```python
from build123d import *

# Parameters (mm, degrees)
SKETCH1_R           = 4.45
BOSS_EXTRUDE1_DEPTH = 5.6
CHAMFER1_SIZE       = 0.6


with BuildPart() as part:
    # Sketch1 → Boss-Extrude1 (new body)
    with BuildSketch(Plane(origin=(0, 0, 0), x_dir=(1, 0, 0), z_dir=(0, 1, 0))):
        with BuildLine():
            Line((6, 10.392304845), (-6, 10.392304845))
            ThreePointArc((-6, 10.392304845), (-12, 0), (-6, -10.392304845))
            Line((-6, -10.392304845), (6, -10.392304845))
            ThreePointArc((6, -10.392304845), (12, 0), (6, 10.392304845))
        make_face()
        Circle(SKETCH1_R, mode=Mode.SUBTRACT)
    extrude(amount=BOSS_EXTRUDE1_DEPTH)

    # Chamfer1
    chamfer1_edges = [part.edges().sort_by_distance(p)[0] for p in [
        (-4.45, 5.6, 0),
    ]]
    chamfer(chamfer1_edges, length=CHAMFER1_SIZE)


solid = part.part
```
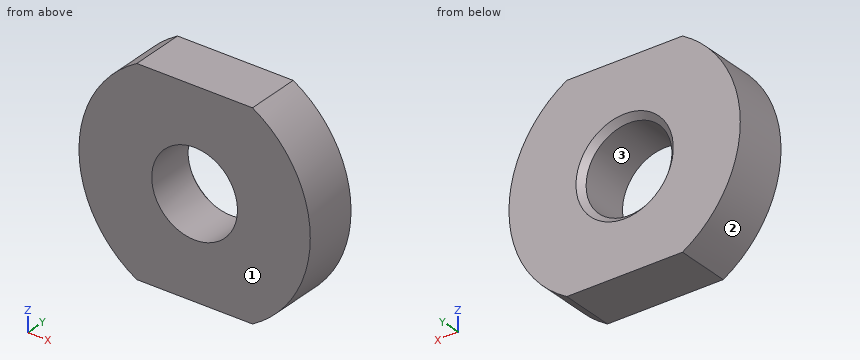
Geometry check sheet. Reference: the model listing, model coordinates, mm. Face numbers are marked on the shaded views. Round coordinates to 2 decimals unless told otherwise and drop trailing zeros. Order: outer loops, then holes, each group sorted by start corner. A loop starts at its lowest first (then second) coordinate and runs counter-clockwise, first axis right, second up. Notation, with made-up numbers: (68.5, -7) -> (96.5, -7) arc R23 cw to (96.5, 8) -> close; hole circle Ø9 at (68.25, -9). An arc over 180 degrees is marked (long way). Return JSON: item names as keys, results as strings. Group by question number.
Q1. Gauge pin test, flat ends, axial feed: pin 1 (1 mm diameter, centred on x = -9.5, z = -7.5, fed in from -Y); pin 2 (1 mm diameter, centred on y = 3, z = -4.5, fed in from -X); pin 3 (1 mm diameter, centred on x = 7.5, y = 4, fed in from -Z). Record the tip position at first contact, or that the pin passes through.
Q2. Section check C-C, the plane y = 0.9. Record the boundary of the cut face in (x, z), plus the area to 3 significant figures.
Q3. Section check A-A, the plane z = 0. Record the boundary of the cut face in (x, y).
Q4. Section check B-B, the plane x = 0. Record the boundary of the cut face in (y, z).
Q5. Material ranges on probe 1 along Z at (x, y) = (0, 3.4); probe 2 along X at (y, z) = (1.1, 0.75); probe 3 along Z at (x, y) = (-1.25, 5.05), recorded low to high. Write a range as from..to.
Q6. Section check D-D, the plane x = 6.5. Record the boundary of the cut face in (y, z), plus the area to 3 significant figures.
Q7. Release check for a two-part mould opening along X. For the marked faces 1, 2 and 3 record: released by +X, released by -X, zero draft, split by the parting line, or undercut.
Numbers:
{
 "1": {"pin 1": "y = 0", "pin 2": "x = -11.31", "pin 3": "z = -9.75"},
 "2": {"outline": "(-6, -10.39) -> (6, -10.39) arc R12 ccw to (6, 10.39) -> (-6, 10.39) arc R12 ccw to start; hole circle Ø8.9 at (0, 0)", "area": "364 mm^2"},
 "3": {"outline": "(-12, 0) -> (-4.45, 0) -> (-4.45, 5) -> (-5.05, 5.6) -> (-12, 5.6) -> close; (4.45, 0) -> (12, 0) -> (12, 5.6) -> (5.05, 5.6) -> (4.45, 5) -> close"},
 "4": {"outline": "(0, -10.39) -> (5.6, -10.39) -> (5.6, -5.05) -> (5, -4.45) -> (0, -4.45) -> close; (0, 4.45) -> (5, 4.45) -> (5.6, 5.05) -> (5.6, 10.39) -> (0, 10.39) -> close"},
 "5": {"probe 1": "-10.39..-4.45, 4.45..10.39", "probe 2": "-11.98..-4.39, 4.39..11.98", "probe 3": "-10.39..-4.32, 4.32..10.39"},
 "6": {"outline": "(0, -10.09) -> (5.6, -10.09) -> (5.6, 10.09) -> (0, 10.09) -> close", "area": "113 mm^2"},
 "7": {"face 1": "zero draft", "face 2": "released by -X", "face 3": "undercut"}
}
